Build history of the part. All positions in model axes, mm. A direction names the side the tool comes from. Round coordinates to 2 decimals unless told otherwise and drop trailing zeros. Write each loop counter-clockwise with the first axis right and the second up, starting at its lowest first coordinate (ties: lowest second). Pieces come first, ordered by that corner, then holes.
1) Saw through at A-A (y = 2.45). Write the cut outline in (x, z), plus the area to 3 significant figures.
2) Wall check: probe 1 along Z at (x, y) = (-2.25, 0.5). Give the ranges that are in metal, low to high.
3) Saw through at B-B (x = -18.5). Write the cut outline in (y, z), plus the area to 3 significant figures.
4) Flat gauge pin, fed straight in: pin 1 (0.6 mm diameter, centred on y = 2.5, z = -0.5, fed in from -X). Where does the tip first touch, or does it go through?
5) Which spindle directions (+Z, -Z, +X, -X, +Y, -Y) get a long thin tool onto all of the face, cutting with end or side? Do faces 1 (the flat face through (-6.35, 3, 39)), 2 (the flat face through (-19.05, 3, 39)), 3 (the flat face through (-12.6, 2.05, -0.5)), 4 (the flat face through (-6.35, 2.7, -0.5)). Say none if no direction does.
Solid Edge part; units mm, degrees
sketch "Sketch1" plane through (0, 0, 0) normal (0, -1, 0) x (1, 0, 0)
  line L0 (-0.127, 0.127) -> (-25.273, 0.127)
  line L1 (-25.273, 0.127) -> (-25.273, 37.973)
  line L2 (-25.273, 37.973) -> (-0.127, 37.973)
  line L3 (-0.127, 37.973) -> (-0.127, 0.127)
extrude "Protrusion1" add sketch "Sketch1" against normal up to surface (2.05 mm away)
sketch "Sketch2" plane through (-9.78, 2.05, 19.05) normal (0, 1, 0) x (1, 0, 0)
  line L0 (-9.27, 20.193) -> (3.43, 20.193)
  line L1 (3.43, 20.193) -> (3.43, 18.923)
  line L2 (9.653, 18.923) -> (3.43, 18.923)
  line L3 (9.653, -18.923) -> (9.653, 18.923)
  line L4 (3.43, -18.923) -> (9.653, -18.923)
  line L5 (3.43, -18.923) -> (3.43, -20.1168)
  line L6 (3.43, -20.1168) -> (-9.27, -20.1168)
  line L7 (-9.27, -20.1168) -> (-9.27, -18.923)
  line L8 (-15.493, -18.923) -> (-9.27, -18.923)
  line L9 (-15.493, 18.923) -> (-15.493, -18.923)
  line L10 (-9.27, 18.923) -> (-15.493, 18.923)
  line L11 (-9.27, 18.923) -> (-9.27, 20.193)
extrude "Protrusion2" add sketch "Sketch2" along normal blind 1.27
Evaluation:
1. outline: (-25.27, 0.13) - (-19.05, 0.13) - (-19.05, -1.14) - (-6.35, -1.14) - (-6.35, 0.13) - (-0.13, 0.13) - (-0.13, 37.97) - (-6.35, 37.97) - (-6.35, 39.17) - (-19.05, 39.17) - (-19.05, 37.97) - (-25.27, 37.97) - close
1. area: 983 mm2
2. probe 1: z = 0.13 to 37.97
3. outline: (0, 0.13) - (2.05, 0.13) - (2.05, -1.14) - (3.32, -1.14) - (3.32, 39.17) - (2.05, 39.17) - (2.05, 37.97) - (0, 37.97) - close
3. area: 129 mm2
4. pin 1: stops at x = -19.05
5. face 1: +Z, +X, +Y, -Y
5. face 2: +Z, -X, +Y, -Y
5. face 3: -Z, +X, -X, -Y
5. face 4: -Z, +X, +Y, -Y
